For this review, take the finished solid that the model builds, in its own axes (mm). Face numbers are marked on the shaded views. A direction names the side the tool comes from. Round coordinates to 2 decimals unless told otherwise and drop trailing zeros. Order: outer loops, then holes, each group sorted by start corner. A loop starts at its lowest first (then second) coordinate and runs counter-clockwise, first axis right, second up. Notation, with made-up numbers: (63.5, 1) -> (105.5, 1) arc R19 cw to (105.5, 29) -> close; hole circle Ø9 at (-34.5, -15). An arc over 180 degrees is marked (long way). Use a Markdown table: item, result. Add a question column.
1) Consider section B-B (z = 3.25). State the section outline as (x, y) points (1 decimal).
2) Consider section D-D (x = 30). State the section outline as (y, z) points.
3) Consider section A-A (y = 25). State the section outline as (x, z) points.
4) Consider section C-C (x = 20). State the section outline as (y, z) points.
5) Machinability: for the marked faces 1 and 2, which of the approach directions +Z, -Z, +X, -X, +Y, -Y give a long, thin tool a straight path to every point of the face, cutting with its end or side? Answer none if there is none.
6) Clearance check with a flat-ended pin moving along its axis: P1, Ø12, axis at x = 18.5, y = 30.5, coming from the +Z side. State where the tip first meets the part, or that it passes through.
7) Wall thickness on line 1 along Y through (x, z) = (20, 1.45); line 2 along Z through (x, y) = (18.25, 4); line 3 along X through (y, z) = (26, 4.5): over which ranges is each line inside the solid? List them lowest first. Write a range as [from, to].
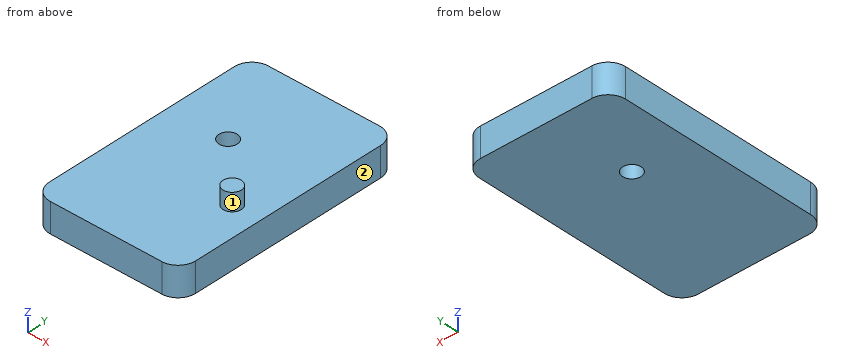
```python
from build123d import *

# Parameters (mm, degrees)
SKETCH_W     = 25
SKETCH_H     = 40
SKETCH_R     = 1.5625
PAD_DEPTH    = 5
FILLET_R     = 3
SKETCH001_R  = 1.56
PAD001_DEPTH = 3


with BuildPart() as part:
    # Sketch → Pad (new body)
    with BuildSketch(Plane.XY):
        with Locations((22.40888, 20)):
            Rectangle(SKETCH_W, SKETCH_H)
        with Locations((20, 25)):
            Circle(SKETCH_R, mode=Mode.SUBTRACT)
    extrude(amount=PAD_DEPTH)

    # Fillet
    fillet_edges = [part.edges().sort_by_distance(p)[0] for p in [
        (9.90888, 0, 2.5),
        (34.90888, 0, 2.5),
        (34.90888, 40, 2.5),
        (9.90888, 40, 2.5),
    ]]
    fillet(fillet_edges, radius=FILLET_R)

    # Sketch001 (on Face7 of Pad) → Pad001 (join)
    with BuildSketch(Plane.XY.offset(5)):
        with Locations((30, 15)):
            Circle(SKETCH001_R)
    extrude(amount=PAD001_DEPTH)


solid = part.part
```
Results list:
| question | item | result |
|---|---|---|
| 1 | outline | (9.9, 3) arc R3 ccw to (12.9, 0) -> (31.9, 0) arc R3 ccw to (34.9, 3) -> (34.9, 37) arc R3 ccw to (31.9, 40) -> (12.9, 40) arc R3 ccw to (9.9, 37) -> close; hole circle Ø3.1 at (20, 25) |
| 2 | outline | (0, 0) -> (40, 0) -> (40, 5) -> (16.56, 5) -> (16.56, 8) -> (13.44, 8) -> (13.44, 5) -> (0, 5) -> close |
| 3 | outline | (9.91, 0) -> (18.44, 0) -> (18.44, 5) -> (9.91, 5) -> close; (21.56, 0) -> (34.91, 0) -> (34.91, 5) -> (21.56, 5) -> close |
| 4 | outline | (0, 0) -> (23.44, 0) -> (23.44, 5) -> (0, 5) -> close; (26.56, 0) -> (40, 0) -> (40, 5) -> (26.56, 5) -> close |
| 5 | face 1 | +Z |
| 5 | face 2 | +Z, -Z, +X, +Y, -Y |
| 6 | P1 | z = 5 |
| 7 | line 1 | [0, 23.44], [26.56, 40] |
| 7 | line 2 | [0, 5] |
| 7 | line 3 | [9.91, 18.8], [21.2, 34.91] |
